Study the drawing (mm; zero at the part's minimum x, y, z) and answer. Give positions to 0.01 mm unless a question says otherwise; leave off trailing zeros. Write each loop counter-clockwise with the first axis right and the second up, starting at its lowest first coordinate (ties: lowest second). Pieces come first, ordered by that corner, then holes.
1) Given pin 1 Ø0.9 at (x, y) = (63, 2) entering from +Z, flat-ended and moving along its own axis, determine where the tip first touches the part or whether it passes through.
2) Find section A-A (z = 22.5). Determine the outline of the cut face in (x, y).
3) Straight lines are drawn through the part: probe 1 along Z at (x, y) = (28, 2.15); probe 2 along Z at (x, y) = (46, 2.85). For each, find the intervals that lie inside material, in ascending order.
4) Find section C-C (x = 19). Determine the outline of the cut face in (y, z).
5) Find section D-D (z = 9). Determine the outline of the cut face in (x, y), plus the area to 3 significant figures.
6) Find section B-B (y = 1.15). Determine the outline of the cut face in (x, z).
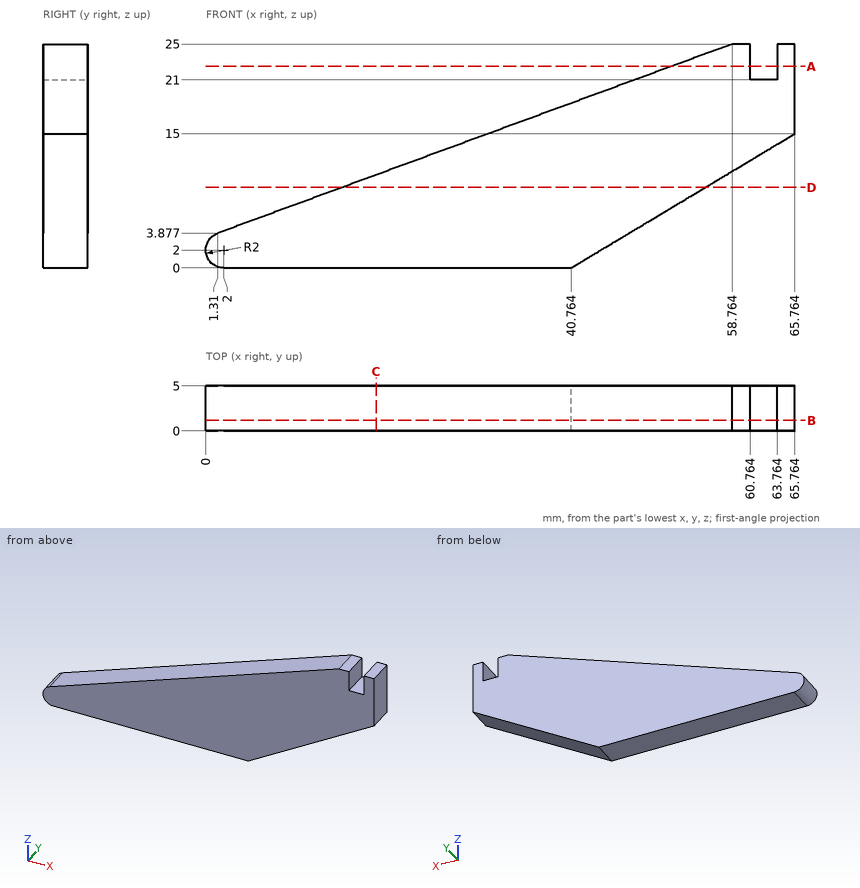
Results:
1. pin 1: stops at z = 21
2. outline: (51.96, 0) - (60.76, 0) - (60.76, 5) - (51.96, 5) - close; (63.76, 0) - (65.76, 0) - (65.76, 5) - (63.76, 5) - close
3. probe 1: z = 0 to 13.69
3. probe 2: z = 3.14 to 20.31
4. outline: (0, 0) - (5, 0) - (5, 10.38) - (0, 10.38) - close
5. outline: (15.24, 0) - (55.76, 0) - (55.76, 5) - (15.24, 5) - close
5. area: 203 mm2
6. outline: (1.31, 3.88) arc R2 ccw to (2, 0) - (40.76, 0) - (65.76, 15) - (65.76, 25) - (63.76, 25) - (63.76, 21) - (60.76, 21) - (60.76, 25) - (58.76, 25) - close
